Print and shaded views of the part. All mm, measured from the part's lowest x, y and z. A direction names the side the tool comes from. Give positions to 0.01 mm unless a question says otherwise; leave off trailing zeros. Order: outer loops, then holes, each group sorted by start corner. A loop starts at its lowest first (then second) coordinate and runs counter-clockwise, first axis right, second up. Notation, with made-up numbers: (88, 85.25) -> (121, 85.25) arc R10 ccw to (121, 91.25) -> close; hole circle Ø8 at (42, -35). An arc over 180 degrees is marked (long way). One line per question, with ' | ' between items. Start each with the question number.
(1) Cut at D-D (x = 30.48). Give the cut face in (y, z).
(2) Cut at B-B (z = 5.08). Give the cut face in (x, y).
(3) Cut at A-A (x = 5.08). Give the cut face in (y, z), then the cut area to 3 significant figures.
(4) Pull direction X, two halves, no side cores. Call the marked faces 4, 5, 6 and 7: +X half, -X half, draft (parallel to the pull), parting line (faces both ways), or undercut.
(5) Drill centre lines: L1, parallel to X at y = 15.24, z = 4; L2, parallel to X at y = 1.55, z = 5.08 (1 decimal); L3, parallel to X at y = 1.4, z = 5.08. Where is each one in solid material? Low to high. Write a range as from..to.
(6) Cut at C-C (y = 23). Give the cut face in (x, z).
(7) Which spindle directions (+Z, -Z, +X, -X, +Y, -Y) get a long thin tool onto all of the face, cutting with end or side? Do the marked faces 1, 2 and 3. Say none if no direction does.
(8) Pin check, flat tips, straight feed: pin 1 Ø1.5 at (x, z) = (33.5, 6.5) entering from +Y; pin 2 Ø5 at (x, z) = (5, 7) entering from +Y; pin 3 Ø3 at (y, z) = (31.5, 8.5) entering from +X (1 decimal); pin 4 Ø4.5 at (x, z) = (55.88, 5.08) entering from +Y. Stop position of each tip, or through.
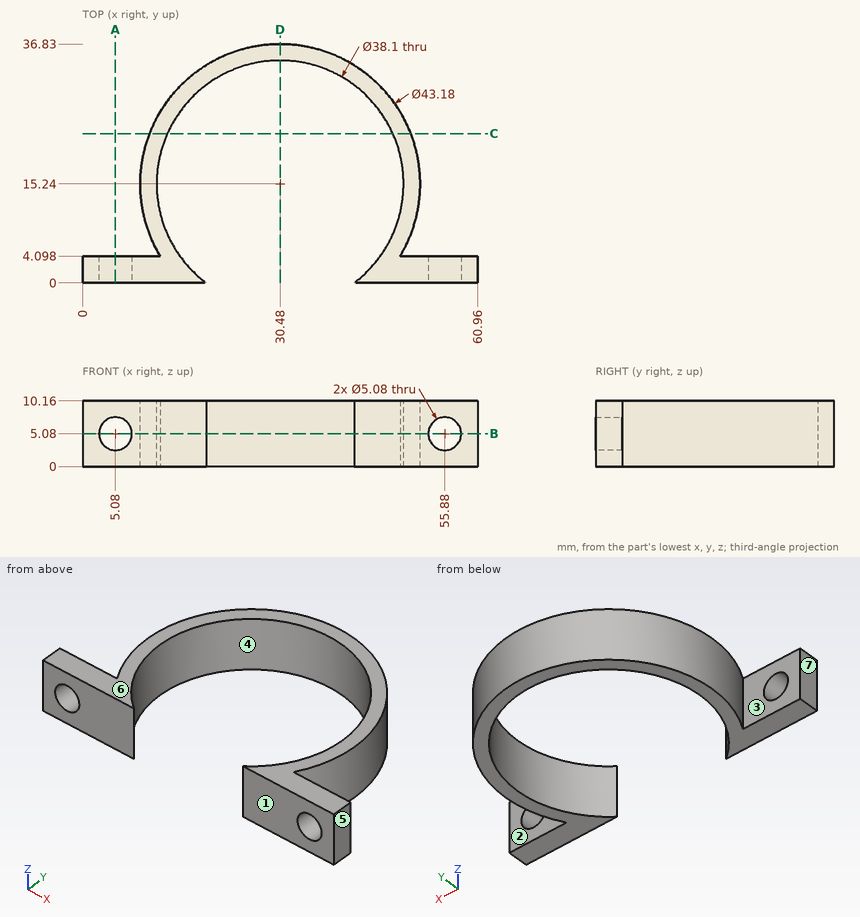
Result set:
1) outline: (34.29, 0) -> (36.83, 0) -> (36.83, 10.16) -> (34.29, 10.16) -> close
2) outline: (0, 0) -> (2.54, 0) -> (2.54, 4.1) -> (0, 4.1) -> close; (7.62, 0) -> (19.05, 0) arc R19.05 cw (long way) to (41.91, 0) -> (53.34, 0) -> (53.34, 4.1) -> (48.97, 4.1) arc R21.59 ccw (long way) to (11.99, 4.1) -> (7.62, 4.1) -> close; (58.42, 0) -> (60.96, 0) -> (60.96, 4.1) -> (58.42, 4.1) -> close
3) outline: (0, 0) -> (4.1, 0) -> (4.1, 2.54) -> (0, 2.54) -> close; (0, 7.62) -> (4.1, 7.62) -> (4.1, 10.16) -> (0, 10.16) -> close | area: 20.8 mm2
4) face 4: undercut | face 5: +X half | face 6: draft | face 7: -X half
5) L1: x = 8.89..11.43, 49.53..52.07 | L2: x = 0..2.5, 7.6..17.2, 43.7..53.3, 58.4..61 | L3: x = 0..2.54, 7.62..17.39, 43.57..53.34, 58.42..60.96
6) outline: (10.33, 0) -> (13.08, 0) -> (13.08, 10.16) -> (10.33, 10.16) -> close; (47.88, 0) -> (50.63, 0) -> (50.63, 10.16) -> (47.88, 10.16) -> close
7) face 1: +Z, -Z, +X, -X, -Y | face 2: +Z, -Z, +X | face 3: +Z, -Z, -X
8) pin 1: stops at y = 36.71 | pin 2: stops at y = 4.1 | pin 3: stops at x = 46.2 | pin 4: passes through
